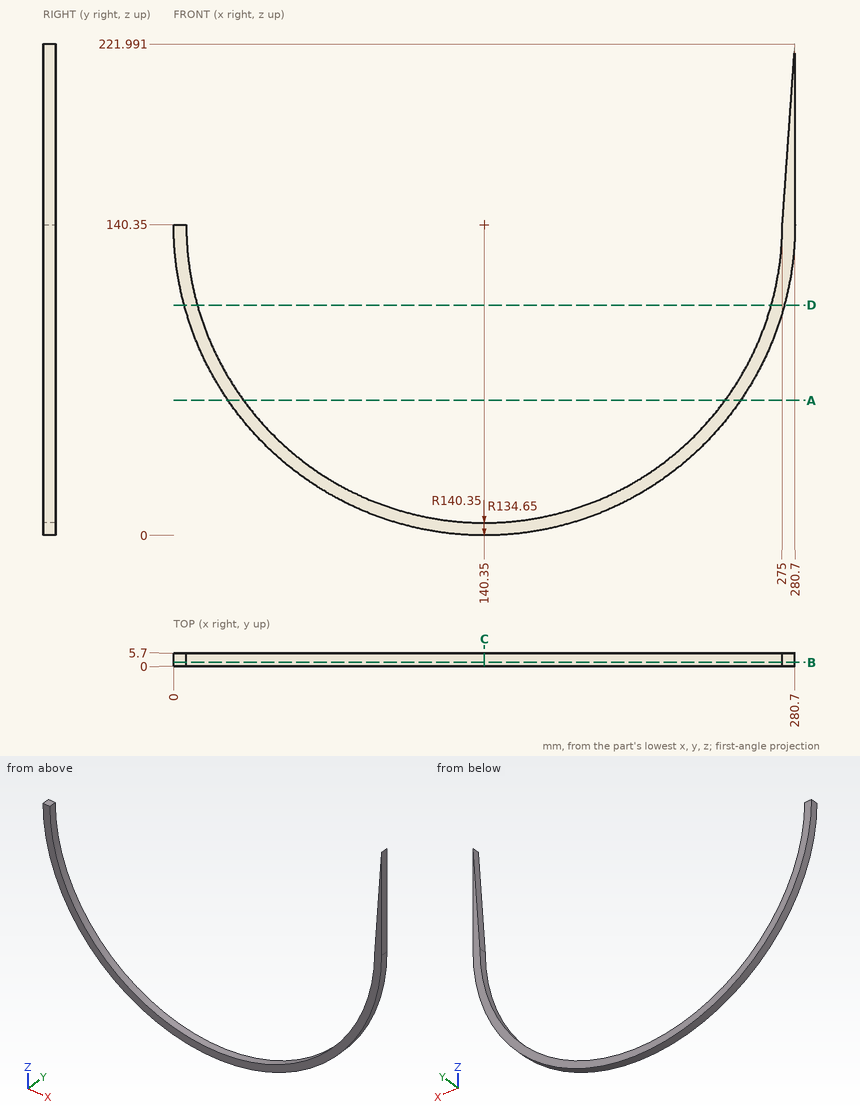
Design review of the part shown in the three views and the two pictorial views. Dimensions are in mm from the part's minimum x, y and z. Give positions to 0.01 mm unless a question says otherwise; leave off trailing zeros. Loops run counter-clockwise (first coordinate to the right, second up) from the corner with the lowest first, then second, coordinate; pieces in that order, holes last. Notation, with made-up numbers: (60.5, 79.5) - (100.5, 79.5) arc R22 ccw to (100.5, 96.5) - close; hole circle Ø8 at (40, 16.5). An arc over 180 degrees is marked (long way). Use CSV: the item, a comma, the result in double quotes. Start each with the question number.
1. Wall thickness on L1, parallel to X at y = 0.5, z = 127; L2, parallel to X at y = 2.5, z = 104.5; L3, parallel to Z at x = 183, y = 1.55: over which ranges is each line inside the solid? List them lowest first.
2. Add section B-B (y = 1.6). State the section outline as (x, z) points.
3. Add section D-D (z = 104). State the section outline as (x, y) points.
4. Add section C-C (x = 140.35). State the section outline as (y, z) points.
5. Insertion check: P1, Ø3, axis at x = 140, y = 2, coming from the +Z side; P2, Ø1.5, axis at x = 145.5, y = 4.5, coming from the +Z side. Each pin has a flat end and moves straight along its axis. Give the tip position at first contact, or say it passes through.
6. Add section A-A (z = 61). State the section outline as (x, y) points (1 decimal), plus the area to 3 significant figures.
Results found:
1,L1,"x = 0.64 to 6.36, 274.34 to 280.06"
1,L2,"x = 4.66 to 10.56, 270.14 to 276.04"
1,L3,"z = 6.64 to 12.63"
2,outline,"(0, 140.35) arc R140.35 ccw to (280.7, 140.35) - (280.7, 221.99) - (275, 140.35) arc R134.65 cw to (5.7, 140.35) - close"
3,outline,"(4.79, 0) - (10.7, 0) - (10.7, 5.7) - (4.79, 5.7) - close; (270, 0) - (275.91, 0) - (275.91, 5.7) - (270, 5.7) - close"
4,outline,"(0, 0) - (5.7, 0) - (5.7, 5.7) - (0, 5.7) - close"
5,P1,"stops at z = 5.71"
5,P2,"stops at z = 5.83"
6,outline,"(24.6, 0) - (31.6, 0) - (31.6, 5.7) - (24.6, 5.7) - close; (249.1, 0) - (256.1, 0) - (256.1, 5.7) - (249.1, 5.7) - close"
6,area,"79.6 mm²"
